```python
from build123d import *
from build123d.topology import SkipClean

# Parameters (mm, degrees)
SKETCH3_W           = 58.1
SKETCH3_H           = 99.8
SKETCH3_R           = 1.1
SKETCH3_R_2         = 0.95
SKETCH3_R_3         = 1.4
BOSS_EXTRUDE1_DEPTH = 2
FILLET1_R           = 5
FILLET2_R           = 3
FILLET3_R           = 10
BOSS_EXTRUDE2_START = 1
SKETCH4_R           = 1.6
SKETCH4_R_2         = 0.95
BOSS_EXTRUDE2_DEPTH = 1
SKETCH5_W           = 38.1
SKETCH5_H           = 61.132694782
CUT_EXTRUDE1_DEPTH  = 63.361145756


with BuildPart() as part:
    # Sketch3 → Boss-Extrude1 (new body)
    with BuildSketch(Plane(origin=(0, 0, 0), x_dir=(1, 0, 0), z_dir=(0, 1, 0))):
        with Locations((0, -5.2)):
            Rectangle(SKETCH3_W, SKETCH3_H)
        with Locations(Location((24.05, -50.1, 0), (0, 0, 270))):
            Circle(SKETCH3_R, mode=Mode.SUBTRACT)
        with Locations(Location((-10.3, -10.3, 0), (0, 0, 270))):
            Circle(SKETCH3_R_2, mode=Mode.SUBTRACT)
        with Locations(Location((13.5, 39.7, 0), (0, 0, 270))):
            Circle(SKETCH3_R, mode=Mode.SUBTRACT)
        with Locations(Location((-13.5, 39.7, 0), (0, 0, 270))):
            Circle(SKETCH3_R, mode=Mode.SUBTRACT)
        with Locations(Location((-24.05, -50.1, 0), (0, 0, 270))):
            Circle(SKETCH3_R, mode=Mode.SUBTRACT)
        with Locations(Location((-24.5, 27.9, 0), (0, 0, 270))):
            Circle(SKETCH3_R_3, mode=Mode.SUBTRACT)
        with Locations(Location((24.5, 27.9, 0), (0, 0, 270))):
            Circle(SKETCH3_R_3, mode=Mode.SUBTRACT)
        with Locations(Location((10.3, 10.3, 0), (0, 0, 270))):
            Circle(SKETCH3_R_2, mode=Mode.SUBTRACT)
        with Locations(Location((10.3, -10.3, 0), (0, 0, 270))):
            Circle(SKETCH3_R_2, mode=Mode.SUBTRACT)
        with Locations(Location((-10.3, 10.3, 0), (0, 0, 270))):
            Circle(SKETCH3_R_2, mode=Mode.SUBTRACT)
        with Locations(Location((-24.5, -30.1, 0), (0, 0, 270))):
            Circle(SKETCH3_R_3, mode=Mode.SUBTRACT)
        with Locations(Location((24.5, -30.1, 0), (0, 0, 270))):
            Circle(SKETCH3_R_3, mode=Mode.SUBTRACT)
        with BuildLine():
            Line((19.05, -45.1), (19.05, -22.090559159))
            Line((19.05, -22.090559159), (8.77972042, -11.82027958))
            ThreePointArc((8.77972042, -11.82027958), (8.77972042, -8.77972042), (11.82027958, -8.77972042))
            Line((11.82027958, -8.77972042), (19.05, -16.009440841))
            Line((19.05, -16.009440841), (19.05, 16.009440841))
            Line((19.05, 16.009440841), (11.82027958, 8.77972042))
            ThreePointArc((11.82027958, 8.77972042), (8.77972042, 8.77972042), (8.77972042, 11.82027958))
            Line((8.77972042, 11.82027958), (19.05, 22.090559159))
            Line((19.05, 22.090559159), (19.05, 34.7))
            Line((19.05, 34.7), (-19.05, 34.7))
            Line((-19.05, 34.7), (-19.05, 22.090559159))
            Line((-19.05, 22.090559159), (-8.77972042, 11.82027958))
            ThreePointArc((-8.77972042, 11.82027958), (-8.77972042, 8.77972042), (-11.82027958, 8.77972042))
            Line((-11.82027958, 8.77972042), (-19.05, 16.009440841))
            Line((-19.05, 16.009440841), (-19.05, -16.009440841))
            Line((-19.05, -16.009440841), (-11.82027958, -8.77972042))
            ThreePointArc((-11.82027958, -8.77972042), (-8.77972042, -8.77972042), (-8.77972042, -11.82027958))
            Line((-8.77972042, -11.82027958), (-19.05, -22.090559159))
            Line((-19.05, -22.090559159), (-19.05, -45.1))
            Line((-19.05, -45.1), (19.05, -45.1))
        make_face(mode=Mode.SUBTRACT)
    extrude(amount=BOSS_EXTRUDE1_DEPTH)

    # Fillet1
    fillet1_edges = [part.edges().sort_by_distance(p)[0] for p in [
        (19.05, 1, -34.7),
        (-19.05, 1, -34.7),
        (-19.05, 1, 45.1),
        (19.05, 1, 45.1),
        (29.05, 1, -44.7),
        (29.05, 1, 55.1),
        (-29.05, 1, 55.1),
        (-29.05, 1, -44.7),
    ]]
    fillet(fillet1_edges, radius=FILLET1_R)

    # Fillet2
    fillet2_edges = [part.edges().sort_by_distance(p)[0] for p in [
        (-19.05, 1, -16.009440841),
        (-19.05, 1, 16.009440841),
        (19.05, 1, 16.009440841),
        (19.05, 1, -16.009440841),
    ]]
    fillet(fillet2_edges, radius=FILLET2_R)

    # Fillet3
    fillet3_edges = [part.edges().sort_by_distance(p)[0] for p in [
        (19.05, 1, -22.090559159),
        (-19.05, 1, -22.090559159),
        (-19.05, 1, 22.090559159),
        (19.05, 1, 22.090559159),
    ]]
    fillet(fillet3_edges, radius=FILLET3_R)

    # Sketch4 → Boss-Extrude2 (add)
    # profile 1 of 4: a face of its own
    with SkipClean():  # the faces are left unmerged after this step: merging them gives an invalid solid
        with BuildSketch(Plane.XZ.offset(BOSS_EXTRUDE2_START)):
            with Locations(Location((-10.3, 10.3, 0), (0, 0, 90))):
                Circle(SKETCH4_R)
            with Locations(Location((-10.3, 10.3, 0), (0, 0, 270))):
                Circle(SKETCH4_R_2, mode=Mode.SUBTRACT)
        # profile 2 of 4: a face of its own
        with BuildSketch(Plane.XZ.offset(BOSS_EXTRUDE2_START)):
            with Locations(Location((10.3, 10.3, 0), (0, 0, 90))):
                Circle(SKETCH4_R)
            with Locations(Location((10.3, 10.3, 0), (0, 0, 270))):
                Circle(SKETCH4_R_2, mode=Mode.SUBTRACT)
        # profile 3 of 4: a face of its own
        with BuildSketch(Plane.XZ.offset(BOSS_EXTRUDE2_START)):
            with Locations(Location((10.3, -10.3, 0), (0, 0, 90))):
                Circle(SKETCH4_R)
            with Locations(Location((10.3, -10.3, 0), (0, 0, 270))):
                Circle(SKETCH4_R_2, mode=Mode.SUBTRACT)
        # profile 4 of 4: a face of its own
        with BuildSketch(Plane.XZ.offset(BOSS_EXTRUDE2_START)):
            with Locations(Location((-10.3, -10.3, 0), (0, 0, 90))):
                Circle(SKETCH4_R)
            with Locations(Location((-10.3, -10.3, 0), (0, 0, 270))):
                Circle(SKETCH4_R_2, mode=Mode.SUBTRACT)
        extrude(amount=-BOSS_EXTRUDE2_DEPTH)

    # Sketch5 → Cut-Extrude1 (cut, through all)
    with BuildSketch(Plane(origin=(0, 2, 0), x_dir=(1, 0, 0), z_dir=(0, 1, 0))):
        with Locations((0, -2.6)):
            Rectangle(SKETCH5_W, SKETCH5_H)
    extrude(amount=-CUT_EXTRUDE1_DEPTH, mode=Mode.SUBTRACT)


solid = part.part
```
The model under review builds one solid part; all positions refer to its coordinate system, in mm. A direction names the side the tool comes from. Round coordinates to 2 decimals unless told otherwise and drop trailing zeros. Order: outer loops, then holes, each group sorted by start corner. A loop starts at its lowest first (then second) coordinate and runs counter-clockwise, first axis right, second up.
(1) Take a section at B-B, the plane z = 33. State the section outline as (x, y) points.
Working result:
outline: (-29.05, 0) - (-19.05, 0) - (-19.05, 2) - (-29.05, 2) - close; (19.05, 0) - (29.05, 0) - (29.05, 2) - (19.05, 2) - close
(2) Take a section at A-A, the plane x = 3. State the section outline as (y, z) points, plus the area to 3 significant figures.
Working result:
outline: (0, -44.7) - (2, -44.7) - (2, -34.7) - (0, -34.7) - close; (0, 45.1) - (2, 45.1) - (2, 55.1) - (0, 55.1) - close
area: 40.0 mm2
(3) Tool access review of faces 1 (the face through (0, 1, 55.1)), 2 (the face through (0, 1, 45.1)): name each direction out of +Z, -Z, +X, -X, +Y, -Y from which nothing blocks a thin tool from reaching the whole face with its end or side.
Working result:
face 1: +Z, +X, -X, +Y, -Y
face 2: +Y, -Y
(4) Take a section at C-C, the plane y = 0.65. Count the separate pieces of the cut face and the enclosed holes in it, plus the area to 3 significant figures.
Working result:
separate pieces: 1
enclosed holes: 9
area: 2,720 mm2
(5) Wall thickness on L1, parallel to X at y = 1.2, z = -27.9; L2, parallel to X at y = 0.9, z = 50.1; L3, parallel to X at y = 1.7, z = -10: over which ranges is each line inside the solid? List them lowest first.
Working result:
L1: x = -29.05 to -25.9, -23.1 to -19.05, 19.05 to 23.1, 25.9 to 29.05
L2: x = -29.05 to -25.15, -22.95 to 22.95, 25.15 to 29.05
L3: x = -29.05 to -19.05, 19.05 to 29.05
(6) Take a section at D-D, the plane z = -27.9. State the section outline as (x, y) points, plus the area to 3 significant figures.
Working result:
outline: (-29.05, 0) - (-25.9, 0) - (-25.9, 2) - (-29.05, 2) - close; (-23.1, 0) - (-19.05, 0) - (-19.05, 2) - (-23.1, 2) - close; (19.05, 0) - (23.1, 0) - (23.1, 2) - (19.05, 2) - close; (25.9, 0) - (29.05, 0) - (29.05, 2) - (25.9, 2) - close
area: 28.8 mm2
(7) Mouldability with a two-part tool opening along X and no side actions: class faces 3 (the face through (0, 1, -44.7)), 4 (the face through (29.05, 1, 6)), 5 (the face through (24, 1, 49)) as released by +X, released by -X, zero draft, split by the parting line, or undercut.
Working result:
face 3: zero draft
face 4: released by +X
face 5: undercut
